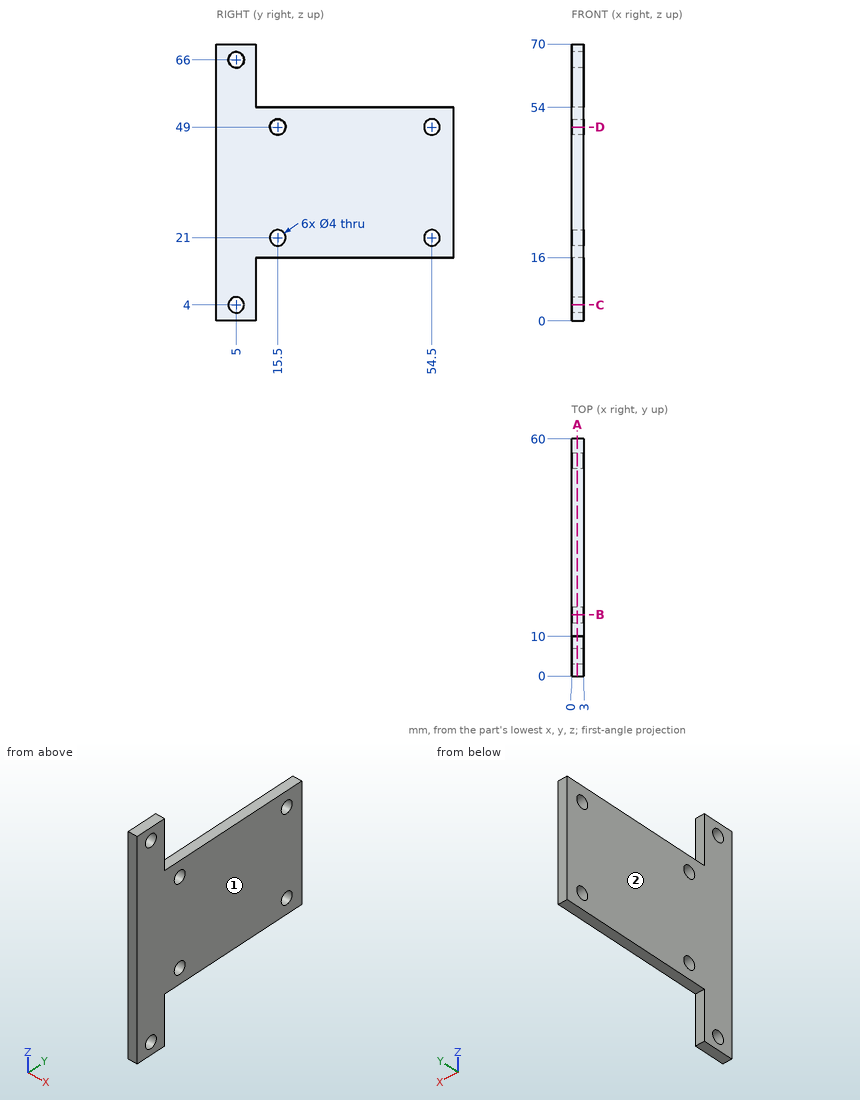
Here's the drawing with two shaded views (mm, measured from the low corner). I have some questions. Give positions to 0.01 mm unless a question says otherwise; leave off trailing zeros. Loops run counter-clockwise (first coordinate to the right, second up) from the corner with the lowest first, then second, coordinate; pieces in that order, holes last. Notation, with made-up numbers: M 86,32 L 123,32 A14 ccw 123,38 Z; hole C 27.25,68 d3. An arc over 180 degrees is marked long. One line per item, written item: value. Start each with the question number.
1) If we section it at A-A, the plane x = 1.45: Write out the boundary of the cut face in (y, z), and give its area (3 significant figures).
2) If I drill on line 1 (Y direction, x = 1.45, z = 49); line 2 (Y direction, x = 1.15, z = 66); line 3 (Z direction, x = 1, y = 53), over which ranges is the centre line in solid material (lowest first)? Write a range as [from, to].
3) Thinking about a two-plate mould opening in X: for the marked faces 1 and 2, which applies, +X half, -X half, draft (parallel to the pull), parting line (faces both ways), or undercut?
4) If we section it at B-B, the plane y = 15.5: Write out the boundary of the cut face in (x, z), and give its area (3 significant figures).
5) I'm going to push flat-ended pins straight in: pin 1 (1.5 mm diameter, centred on x = 1.5, y = 43.5, fed in from -Z); pin 2 (1.5 mm diameter, centred on x = 2, y = 14, fed in from +Z); pin 3 (1.5 mm diameter, centred on x = 1.5, z = 63, fed in from +Y). Where does each tip first touch, or does it pass through?
6) If we section it at D-D, the plane z = 49: Write out the boundary of the cut face in (x, y), and give its area (3 significant figures).
7) If we section it at C-C, the plane z = 4: Write out the boundary of the cut face in (x, y), and give its area (3 significant figures).
Completed:
1. outline: M 0,0 L 10,0 L 10,16 L 60,16 L 60,54 L 10,54 L 10,70 L 0,70 Z; hole C 5,4 d4; hole C 5,66 d4; hole C 15.5,21 d4; hole C 15.5,49 d4; hole C 54.5,21 d4; hole C 54.5,49 d4
1. area: 2,520 mm^2
2. line 1: y = [0, 13.5], [17.5, 52.5], [56.5, 60]
2. line 2: y = [0, 3], [7, 10]
2. line 3: z = [16, 19.68], [22.32, 47.68], [50.32, 54]
3. face 1: +X half
3. face 2: -X half
4. outline: M 0,16 L 3,16 L 3,19 L 0,19 Z; M 0,23 L 3,23 L 3,47 L 0,47 Z; M 0,51 L 3,51 L 3,54 L 0,54 Z
4. area: 90.0 mm^2
5. pin 1: stops at z = 16
5. pin 2: stops at z = 54
5. pin 3: stops at y = 10
6. outline: M 0,0 L 3,0 L 3,13.5 L 0,13.5 Z; M 0,17.5 L 3,17.5 L 3,52.5 L 0,52.5 Z; M 0,56.5 L 3,56.5 L 3,60 L 0,60 Z
6. area: 156 mm^2
7. outline: M 0,0 L 3,0 L 3,3 L 0,3 Z; M 0,7 L 3,7 L 3,10 L 0,10 Z
7. area: 18.0 mm^2
